Model file for the job. Use its own axes, mm. Face numbers are marked on the shaded views. A direction names the side the tool comes from. Give positions to 0.01 mm unless a question says otherwise; leave off trailing zeros. Write each loop counter-clockwise with the first axis right and the second up, starting at its lowest first coordinate (ties: lowest second). Pieces come first, ordered by that corner, then holes.
```python
from build123d import *

# Parameters (mm, degrees)
SKETCH1_W               = 80
SKETCH1_H               = 80
BOSS_EXTRUDE1_DEPTH     = 80
SHELL1_T                = -3
CUT_EXTRUDE1_REACH      = 140.564
SKETCH2_R               = 27
SKETCH3_R               = 30
SKETCH3_R_2             = 27
BOSS_EXTRUDE2_DEPTH     = 9
BOSS_EXTRUDE3_DEPTH     = 3
SKETCH5_W               = 104.199084268
SKETCH5_H               = 10
CUT_EXTRUDE2_DEPTH      = 139.564064606
CUT_EXTRUDE2_DEPTH_BACK = 139.564064606
BOSS_EXTRUDE4_DEPTH     = 3
FILLET3_R               = 3
FILLET4_R               = 2
CUT_EXTRUDE5_REACH      = 129.138
SKETCH9_R               = 2
SKETCH13_W              = 80
SKETCH13_H              = 60
BOSS_EXTRUDE6_DEPTH     = 70
SKETCH14_W              = 74
SKETCH14_H              = 60
CUT_EXTRUDE8_DEPTH      = 67
SKETCH15_W              = 80
SKETCH15_H              = 140
SKETCH15_W_2            = 74
SKETCH15_H_2            = 134
BOSS_EXTRUDE7_DEPTH     = 20
SKETCH12_R              = 28
CUT_EXTRUDE7_DEPTH      = 12
FILLET5_R               = 3
SKETCH16_W              = 9.113547255
SKETCH16_H              = 9.484027798
SKETCH16_W_2            = 8
SKETCH16_H_2            = 8
BOSS_EXTRUDE8_DEPTH     = 10
SKETCH17_W              = 10
SKETCH17_H              = 114
CUT_EXTRUDE9_DEPTH      = 181
CUT_EXTRUDE10_START     = -10
SKETCH18_W              = 54
SKETCH18_H              = 10
CUT_EXTRUDE10_DEPTH     = 171
FILLET6_R               = 3
CUT_EXTRUDE11_REACH     = 186.662
SKETCH19_R              = 2
FILLET7_R               = 3
CUT_EXTRUDE12_REACH     = 182
SKETCH20_W              = 20
SKETCH20_H              = 15


with BuildPart() as part:
    # Sketch1 → Boss-Extrude1 (new body)
    with BuildSketch(Plane(origin=(0, 0, 0), x_dir=(1, 0, 0), z_dir=(0, 1, 0))):
        with Locations((40, 40)):
            Rectangle(SKETCH1_W, SKETCH1_H)
    extrude(amount=BOSS_EXTRUDE1_DEPTH)

    # Shell1
    shell1_openings = [part.faces().sort_by_distance(p)[0] for p in [
        (40, 40, 0),
    ]]
    offset(amount=SHELL1_T, openings=shell1_openings, kind=Kind.INTERSECTION)

    # Sketch2 → Cut-Extrude1 (cut, up to next)
    with BuildSketch(Plane(origin=(0, 0, -80), x_dir=(-1, 0, 0), z_dir=(0, 0, -1)), mode=Mode.PRIVATE) as cut_extrude1_sk1:
        with Locations((-40, 40)):
            Circle(SKETCH2_R)
    cut_extrude1_tool1 = extrude(cut_extrude1_sk1.sketch, amount=-CUT_EXTRUDE1_REACH, mode=Mode.PRIVATE) & part.part
    add(cut_extrude1_tool1.solids().sort_by_distance((40, 40, -80))[0], mode=Mode.SUBTRACT)

    # Sketch3 → Boss-Extrude2 (add)
    with BuildSketch(Plane.XY.offset(-77)):
        with Locations((40, 40)):
            Circle(SKETCH3_R)
        with Locations(Location((40, 40, 0), (0, 0, 180))):
            Circle(SKETCH3_R_2, mode=Mode.SUBTRACT)
    extrude(amount=BOSS_EXTRUDE2_DEPTH)

    # Sketch4 → Boss-Extrude3 (add)
    with BuildSketch(Plane.XY.offset(-68)):
        with BuildLine():
            Line((18, 60.396078054), (18, 19.603921946))
            ThreePointArc((18, 19.603921946), (10, 40), (18, 60.396078054))
        make_face()
        with BuildLine():
            Line((62, 60.396078054), (62, 19.603921946))
            ThreePointArc((62, 19.603921946), (70, 40), (62, 60.396078054))
        make_face()
    extrude(amount=BOSS_EXTRUDE3_DEPTH)

    # Sketch5 → Cut-Extrude2 (cut, two sides)
    with BuildSketch(Plane.XZ) as cut_extrude2_sk:
        with Locations((52.099542134, -5)):
            Rectangle(SKETCH5_W, SKETCH5_H)
    extrude(amount=CUT_EXTRUDE2_DEPTH, mode=Mode.SUBTRACT)
    extrude(cut_extrude2_sk.sketch, amount=-CUT_EXTRUDE2_DEPTH_BACK, mode=Mode.SUBTRACT)

    # Sketch8 → Boss-Extrude4 (add)
    with BuildSketch(Plane.XY.offset(-68)):
        with BuildLine():
            Line((18, 60.396078054), (18, 52.135192758))
            Line((18, 52.135192758), (62, 52.135192758))
            Line((62, 52.135192758), (62, 60.396078054))
            ThreePointArc((62, 60.396078054), (40, 70), (18, 60.396078054))
        make_face()
    extrude(amount=BOSS_EXTRUDE4_DEPTH)

    # Fillet3
    fillet3_edges = [part.edges().sort_by_distance(p)[0] for p in [
        (18, 52.135192758, -66.5),
        (62, 52.135192758, -66.5),
    ]]
    fillet(fillet3_edges, radius=FILLET3_R)

    # Fillet4
    fillet4_edges = [part.edges().sort_by_distance(p)[0] for p in [
        (40, 70, -65),
    ]]
    fillet(fillet4_edges, radius=FILLET4_R)

    # Sketch9 → Cut-Extrude5 (cut, up to next)
    with BuildSketch(Plane(origin=(0, 0, -68), x_dir=(-1, 0, 0), z_dir=(0, 0, -1)), mode=Mode.PRIVATE) as cut_extrude5_sk1:
        with Locations((-52, 57.5)):
            Circle(SKETCH9_R)
    cut_extrude5_tool1 = extrude(cut_extrude5_sk1.sketch, amount=-CUT_EXTRUDE5_REACH, mode=Mode.PRIVATE) & part.part
    # Sketch9 → Cut-Extrude5 (cut, up to next)
    with BuildSketch(Plane(origin=(0, 0, -68), x_dir=(-1, 0, 0), z_dir=(0, 0, -1)), mode=Mode.PRIVATE) as cut_extrude5_sk2:
        with Locations((-28, 57.5)):
            Circle(SKETCH9_R)
    cut_extrude5_tool2 = extrude(cut_extrude5_sk2.sketch, amount=-CUT_EXTRUDE5_REACH, mode=Mode.PRIVATE) & part.part
    add(cut_extrude5_tool1.solids().sort_by_distance((52, 57.5, -68))[0], mode=Mode.SUBTRACT)
    add(cut_extrude5_tool2.solids().sort_by_distance((28, 57.5, -68))[0], mode=Mode.SUBTRACT)

    # Sketch13 → Boss-Extrude6 (add)
    with BuildSketch(Plane(origin=(0, 0, -80), x_dir=(-1, 0, 0), z_dir=(0, 0, -1))):
        with Locations((-40, 110)):
            Rectangle(SKETCH13_W, SKETCH13_H)
    extrude(amount=-BOSS_EXTRUDE6_DEPTH)

    # Sketch14 → Cut-Extrude8 (cut)
    with BuildSketch(Plane.XY.offset(-10)):
        with Locations((40, 107)):
            Rectangle(SKETCH14_W, SKETCH14_H)
    extrude(amount=-CUT_EXTRUDE8_DEPTH, mode=Mode.SUBTRACT)

    # Sketch15 → Boss-Extrude7 (add)
    with BuildSketch(Plane.XY.offset(-10)):
        with Locations((40, 70)):
            Rectangle(SKETCH15_W, SKETCH15_H)
        with Locations((40, 70)):
            Rectangle(SKETCH15_W_2, SKETCH15_H_2, mode=Mode.SUBTRACT)
    extrude(amount=BOSS_EXTRUDE7_DEPTH)

    # Sketch12 → Cut-Extrude7 (cut)
    with BuildSketch(Plane(origin=(0, 0, -80), x_dir=(-1, 0, 0), z_dir=(0, 0, -1))):
        with Locations((-40, 40)):
            Circle(SKETCH12_R)
    extrude(amount=-CUT_EXTRUDE7_DEPTH, mode=Mode.SUBTRACT)

    # Fillet5
    fillet5_edges = [part.edges().sort_by_distance(p)[0] for p in [
        (80, 140, -45),
        (0, 140, -45),
        (3, 137, -43.5),
        (77, 137, -43.5),
        (3, 3, -43.5),
        (77, 3, -43.5),
        (0, 0, -45),
        (80, 0, -45),
    ]]
    fillet(fillet5_edges, radius=FILLET5_R)

    # Sketch16 → Boss-Extrude8 (add)
    with BuildSketch(Plane.XY.offset(10)):
        with Locations((6.443226372, 6.257986101)):
            Rectangle(SKETCH16_W, SKETCH16_H)
        with Locations((73, 7)):
            Rectangle(SKETCH16_W_2, SKETCH16_H_2)
        with Locations((73, 133)):
            Rectangle(SKETCH16_W_2, SKETCH16_H_2)
        with Locations((7, 133)):
            Rectangle(SKETCH16_W_2, SKETCH16_H_2)
    extrude(amount=-BOSS_EXTRUDE8_DEPTH)

    # Sketch17 → Cut-Extrude9 (cut, through all)
    with BuildSketch(Plane.ZY):
        with Locations((-13, 70)):
            Rectangle(SKETCH17_W, SKETCH17_H)
    extrude(amount=-CUT_EXTRUDE9_DEPTH, mode=Mode.SUBTRACT)

    # Sketch18 → Cut-Extrude10 (cut, through all)
    with BuildSketch(Plane(origin=(0, 140, 0), x_dir=(1, 0, 0), z_dir=(0, 1, 0)).offset(CUT_EXTRUDE10_START)):
        with Locations((40, 13)):
            Rectangle(SKETCH18_W, SKETCH18_H)
    extrude(amount=-CUT_EXTRUDE10_DEPTH, mode=Mode.SUBTRACT)

    # Fillet6
    fillet6_edges = [part.edges().sort_by_distance(p)[0] for p in [
        (1.5, 13, -18),
        (1.5, 127, -18),
        (1.5, 127, -8),
        (1.5, 13, -8),
        (78.5, 13, -18),
        (78.5, 127, -18),
        (78.5, 127, -8),
        (78.5, 13, -8),
        (13, 1.5, -8),
        (13, 1.5, -18),
        (67, 1.5, -18),
        (67, 1.5, -8),
    ]]
    fillet(fillet6_edges, radius=FILLET6_R)

    # Sketch19 → Cut-Extrude11 (cut, up to next)
    with BuildSketch(Plane.XY.offset(10), mode=Mode.PRIVATE) as cut_extrude11_sk1:
        with Locations((5.5, 134.5)):
            Circle(SKETCH19_R)
    cut_extrude11_tool1 = extrude(cut_extrude11_sk1.sketch, amount=-CUT_EXTRUDE11_REACH, mode=Mode.PRIVATE) & part.part
    # Sketch19 → Cut-Extrude11 (cut, up to next)
    with BuildSketch(Plane.XY.offset(10), mode=Mode.PRIVATE) as cut_extrude11_sk2:
        with Locations((74.5, 134.5)):
            Circle(SKETCH19_R)
    cut_extrude11_tool2 = extrude(cut_extrude11_sk2.sketch, amount=-CUT_EXTRUDE11_REACH, mode=Mode.PRIVATE) & part.part
    # Sketch19 → Cut-Extrude11 (cut, up to next)
    with BuildSketch(Plane.XY.offset(10), mode=Mode.PRIVATE) as cut_extrude11_sk3:
        with Locations((74.5, 5.5)):
            Circle(SKETCH19_R)
    cut_extrude11_tool3 = extrude(cut_extrude11_sk3.sketch, amount=-CUT_EXTRUDE11_REACH, mode=Mode.PRIVATE) & part.part
    # Sketch19 → Cut-Extrude11 (cut, up to next)
    with BuildSketch(Plane.XY.offset(10), mode=Mode.PRIVATE) as cut_extrude11_sk4:
        with Locations((5.5, 5.5)):
            Circle(SKETCH19_R)
    cut_extrude11_tool4 = extrude(cut_extrude11_sk4.sketch, amount=-CUT_EXTRUDE11_REACH, mode=Mode.PRIVATE) & part.part
    add(cut_extrude11_tool1.solids().sort_by_distance((5.5, 134.5, 10))[0], mode=Mode.SUBTRACT)
    add(cut_extrude11_tool2.solids().sort_by_distance((74.5, 134.5, 10))[0], mode=Mode.SUBTRACT)
    add(cut_extrude11_tool3.solids().sort_by_distance((74.5, 5.5, 10))[0], mode=Mode.SUBTRACT)
    add(cut_extrude11_tool4.solids().sort_by_distance((5.5, 5.5, 10))[0], mode=Mode.SUBTRACT)

    # Fillet7
    fillet7_edges = [part.edges().sort_by_distance(p)[0] for p in [
        (11, 11, 5),
        (69, 11, 5),
        (69, 129, 5),
        (11, 129, 5),
    ]]
    fillet(fillet7_edges, radius=FILLET7_R)

    # Sketch20 → Cut-Extrude12 (cut, up to next)
    with BuildSketch(Plane(origin=(0, 140, 0), x_dir=(1, 0, 0), z_dir=(0, 1, 0)), mode=Mode.PRIVATE) as cut_extrude12_sk1:
        with Locations((40, 15.5)):
            Rectangle(SKETCH20_W, SKETCH20_H)
    cut_extrude12_tool1 = extrude(cut_extrude12_sk1.sketch, amount=-CUT_EXTRUDE12_REACH, mode=Mode.PRIVATE) & part.part
    add(cut_extrude12_tool1.solids().sort_by_distance((40, 140, -15.5))[0], mode=Mode.SUBTRACT)


solid = part.part
```
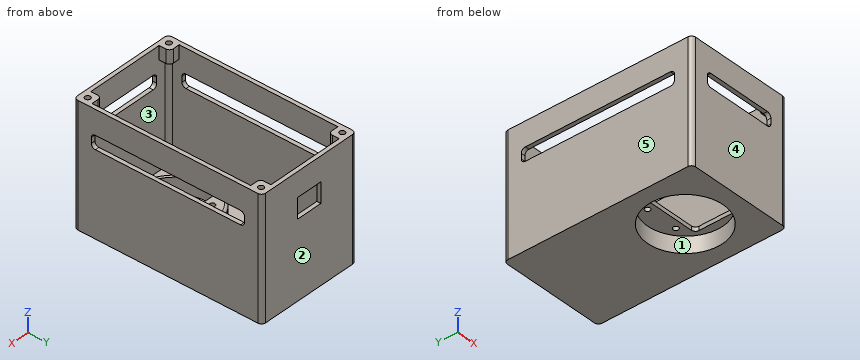
1. Pin check, flat tips, straight feed: P1, Ø10, axis at x = 37.5, y = 96.5, coming from the +Z side; P2, Ø1.5, axis at y = 1.5, z = -12, coming from the +X side; P3, Ø1.5, axis at x = 79, z = -13, coming from the +Y side. Stop position of each tip, or through.
Calculated:
P1: stops at z = -77
P2: stops at x = 79.9
P3: stops at y = 139.73
2. Slice it at A-A, the plane z = -69.5. Write the cut outline in (x, y).
Calculated:
outline: (0, 3) arc R3 ccw to (3, 0) - (77, 0) arc R3 ccw to (80, 3) - (80, 137) arc R3 ccw to (77, 140) - (3, 140) arc R3 ccw to (0, 137) - close; circle Ø60 at (40, 40); hole (3, 6) arc R3 ccw to (6, 3) - (74, 3) arc R3 ccw to (77, 6) - (77, 134) arc R3 ccw to (74, 137) - (6, 137) arc R3 ccw to (3, 134) - close; hole circle Ø56 at (40, 40)
3. Slice it at C-C, the plane y = 78. Write the cut outline in (x, z).
Calculated:
outline: (0, -80) - (80, -80) - (80, -18) - (77, -18) - (77, -77) - (3, -77) - (3, -18) - (0, -18) - close; (0, -8) - (3, -8) - (3, 10) - (0, 10) - close; (77, -8) - (80, -8) - (80, 10) - (77, 10) - close
4. Which spindle directions (+Z, -Z, +X, -X, +Y, -Y) get a long thin tool onto all of the face, cutting with end or side? Do the marked faces 1 and 2. Say none if no direction does.
Calculated:
face 1: -Z
face 2: +Z, -Z, +X, -X, +Y
5. Slice it at D-D, the plane z = -2.5. Write the cut outline in (x, y).
Calculated:
outline: (0, 3) arc R3 ccw to (3, 0) - (77, 0) arc R3 ccw to (80, 3) - (80, 137) arc R3 ccw to (77, 140) - (3, 140) arc R3 ccw to (0, 137) - close; hole (3, 6) arc R3 ccw to (6, 3) - (74, 3) arc R3 ccw to (77, 6) - (77, 134) arc R3 ccw to (74, 137) - (6, 137) arc R3 ccw to (3, 134) - close
6. Pull direction Y, two halves, no side cores. Call the marked faces 3, 4 and 5: +Y half, -Y half, draft (parallel to the pull), parting line (faces both ways), or undercut.
Calculated:
face 3: undercut
face 4: -Y half
face 5: draft
7. Slice it at B-B, the plane x = 40. Write the cut outline in (y, z).
Calculated:
outline: (0, -80) - (12, -80) - (12, -68) - (10, -68) - (10, -77) - (3, -77) - (3, -18) - (0, -18) - close; (0, -8) - (3, -8) - (3, 10) - (0, 10) - close; (52.14, -68) - (68, -68) - (68, -80) - (140, -80) - (140, -23) - (137, -23) - (137, -77) - (70, -77) - (70, -67) arc R2 ccw to (68, -65) - (52.14, -65) - close; (137, -8) - (140, -8) - (140, 10) - (137, 10) - close
8. Probe probe 1 along Y at (x, z) = (74.5, 7.25); probe 2 along X at (y, z) = (134.5, 3.5); probe 3 along Y at (x, z) = (74, -32). List the from-to ranges inside material, lowest first.
Calculated:
probe 1: y = 0 to 3.5, 7.5 to 11, 129 to 132.5, 136.5 to 140
probe 2: x = 0 to 3.5, 7.5 to 11, 69 to 72.5, 76.5 to 80
probe 3: y = 0 to 3, 137 to 140
